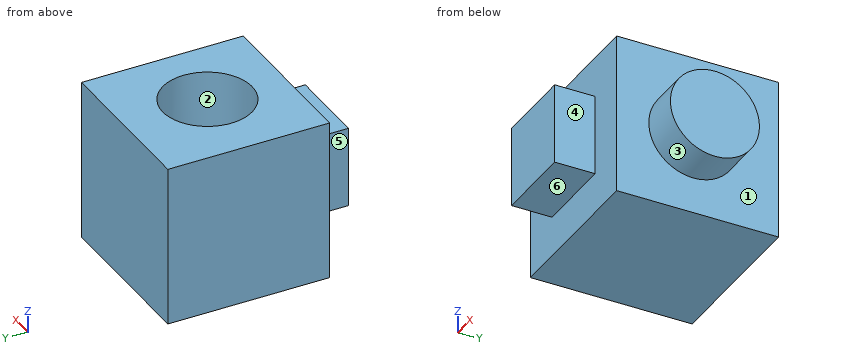
```python
from build123d import *

# Parameters (mm, degrees)
F0_W     = 50.8
F0_H     = 50.8
F1_DEPTH = 50.8
F2_W     = 25.4
F2_H     = 25.4
F3_DEPTH = 12.7
F4_R     = 14.017658
F5_DEPTH = 25.4
F6_R     = 13.98609
F7_DEPTH = 12.7


with BuildPart() as f1:
    # F0 (on Front) → F1 (new body)
    with BuildSketch(Plane.XZ):
        with Locations((-25.4, 25.4)):
            Rectangle(F0_W, F0_H)
    extrude(amount=F1_DEPTH)

    # F2 (on face) → F3 (join)
    with BuildSketch(Plane.XZ.offset(50.8)):
        with Locations((-25.4, 25.4)):
            Rectangle(F2_W, F2_H)
    extrude(amount=F3_DEPTH)

    # F4 (on face) → F5 (cut)
    with BuildSketch(Plane.XY.offset(50.8)):
        with Locations((-24.082342, -26.685146)):
            Circle(F4_R)
    extrude(amount=-F5_DEPTH, mode=Mode.SUBTRACT)

    # F6 (on face) → F7 (join)
    with BuildSketch(Plane.YZ):
        with Locations((-26.733652, 25.350569)):
            Circle(F6_R)
    extrude(amount=F7_DEPTH)


solid = f1.part
```
Geometry check sheet. Reference: the model listing, model coordinates, mm. Face numbers are marked on the shaded views. A direction names the side the tool comes from. Coordinates: 2 decimals unless noted, no trailing zeros. Loops run counter-clockwise (first coordinate to the right, second up) from the corner with the lowest first, then second, coordinate; pieces in that order, holes last.
Item 1: Access from +Z, -Z, +X, -X, +Y, -Y to the whole of each face (thin tool, end or side, straight path). Record for the marked faces 4, 5 and 6.
Item 2: Thickness scan on line 1 (Z direction, x = -30.5, y = -22); line 2 (Y direction, x = -25.5, z = 27.5); line 3 (Y direction, x = -10.5, z = 17). Record the ranges inside material, lowest first.
Item 3: Sectioned sample at D-D, the plane z = 43. Record the boundary of the cut face in (x, y), then the cut area to 3 significant figures.
Item 4: Go/stop test with flat-tipped pins: pin 1 Ø1.5 at (x, z) = (-25.5, 5.5) entering from -Y; pin 2 Ø1 at (x, z) = (2.5, 22.5) entering from -Y; pin 3 Ø10 at (y, z) = (-54, 23) entering from +X. Record where each tip stops, or that it passes through.
Item 5: Sectioned sample at C-C, the plane x = -8.5. Record the boundary of the cut face in (y, z), then the cut area to 3 significant figures.
Item 6: Sectioned sample at B-B, the plane z = 21. Record the boundary of the cut face in (x, y).
Item 7: Release check for a two-part mould opening along X. For the marked faces 1, 2 and 3 record: released by +X, released by -X, zero draft, split by the parting line, or undercut.
Item 8: Sectioned sample at A-A, the plane y = -30.5. Record the boundary of the cut face in (x, z).
Check result:
1. face 4: +Z, -Z, +X, -Y
1. face 5: +Z, -Z, -X, -Y
1. face 6: -Z, +X, -X, -Y
2. line 1: z = 0 to 25.4
2. line 2: y = -63.5 to -40.63, -12.74 to 0
2. line 3: y = -50.8 to 0
3. outline: (-50.8, -50.8) - (0, -50.8) - (0, 0) - (-50.8, 0) - close; hole circle Ø28.04 at (-24.08, -26.69)
3. area: 1,960 mm2
4. pin 1: stops at y = -50.8
4. pin 2: stops at y = -40.52
4. pin 3: stops at x = 0
5. outline: (-50.8, 0) - (0, 0) - (0, 50.8) - (-50.8, 50.8) - close
5. area: 2,580 mm2
6. outline: (-50.8, -50.8) - (-38.1, -50.8) - (-38.1, -63.5) - (-12.7, -63.5) - (-12.7, -50.8) - (0, -50.8) - (0, -40.03) - (12.7, -40.03) - (12.7, -13.44) - (0, -13.44) - (0, 0) - (-50.8, 0) - close
7. face 1: released by +X
7. face 2: undercut
7. face 3: zero draft
8. outline: (-50.8, 0) - (0, 0) - (0, 11.88) - (12.7, 11.88) - (12.7, 38.82) - (0, 38.82) - (0, 50.8) - (-10.59, 50.8) - (-10.59, 25.4) - (-37.57, 25.4) - (-37.57, 50.8) - (-50.8, 50.8) - close
